Autodesk Inventor part; units mm, degrees
ref_plane "YZ Plane" through (0, 0, 0) normal (1, 0, 0) x (0, 1, 0)
ref_plane "XZ Plane" through (0, 0, 0) normal (0, 1, 0) x (-1, 0, 0)
ref_plane "XY Plane" through (0, 0, 0) normal (0, 0, 1) x (1, 0, 0)
sketch "스케치1" plane through (0, 0, 0) normal (0, 1, 0) x (-1, 0, 0)
  circle A0 centre (0, 0) radius 11
  circle A1 centre (0, -8) radius 1.1
  circle A2 centre (0, 0) radius 11
  circle A3 centre (8, 0) radius 1.1
  circle A4 centre (0, 0) radius 11
  circle A5 centre (0, 8) radius 1.1
  circle A6 centre (0, 0) radius 11
  circle A7 centre (-8, 0) radius 1.1
  line L0 (-11, 0) -> (-11, -150)
  line L1 (-11, -150) -> (11, -150)
  line L2 (11, -150) -> (11, 0)
  line L3 (16, -150) -> (-16, -150)
  line L4 (-16, -150) -> (-16, -50)
  line L5 (-16, -50) -> (16, -50)
  line L6 (16, -50) -> (16, -150)
  arc A8 (-11, 0) -> (11, 0) centre (0, 0) ccw
  circle A9 centre (0, 0) radius 4.5
  line L7 (25, -150) -> (-25, -150)
  line L8 (-25, -150) -> (-25, -60)
  line L9 (-25, -60) -> (25, -60)
  line L10 (25, -60) -> (25, -150)
  line L11 (16, -63.3333) -> (21, -63.3333)
  line L12 (21, -63.3333) -> (21, -103.3333)
  line L13 (21, -103.3333) -> (16, -103.3333)
  line L14 (16, -103.3333) -> (16, -63.3333)
  line L15 (16, -106.6667) -> (21, -106.6667)
  line L16 (21, -106.6667) -> (21, -146.6667)
  line L17 (21, -146.6667) -> (16, -146.6667)
  line L18 (16, -146.6667) -> (16, -106.6667)
  line L19 (-16, -63.3333) -> (-21, -63.3333)
  line L20 (-21, -63.3333) -> (-21, -103.3333)
  line L21 (-21, -103.3333) -> (-16, -103.3333)
  line L22 (-16, -103.3333) -> (-16, -63.3333)
  line L23 (-16, -106.6667) -> (-21, -106.6667)
  line L24 (-21, -106.6667) -> (-21, -146.6667)
  line L25 (-21, -146.6667) -> (-16, -146.6667)
  line L26 (-16, -146.6667) -> (-16, -106.6667)
  dimension "d1" = 2.2
  dimension "d5" = 360
  dimension "d7" = 150
  dimension "d8" = 32
  dimension "d9" = 100
  dimension "d24" = 9
  dimension "d26" = 50
  dimension "d27" = 90
  dimension "d28" = 9
  dimension "d29" = 5
  dimension "d30" = 40
  dimension "d31" = 5
  dimension "d32" = 40
  dimension "d33" = 3.3333
  dimension "d34" = 3.3333
  dimension "d35" = 5
  dimension "d36" = 40
  dimension "d37" = 5
  dimension "d38" = 40
  dimension "d39" = 3.3333
  dimension "d40" = 3.3333
extrude "돌출1" add sketch "스케치1" along normal blind 5 contours A0 | L2 L5 L0 A0 | L5 L6 L9 L2 | L2 L9 L0 L5 | L0 L9 L4 L5 | L9 L6 L3 L2 | L2 L1 L0 L9 | L0 L3 L4 L9 | L9 L10 L7 L6 L17 L16 L15 L13 L12 L11 | L4 L19 L20 L21 L23 L24 L25 L7 L8 L9
fillet "모깎기1" radius 2 18 edges at (16, 5, -83.3333) (16, 5, -126.6667) (16, 0, -126.6667) (16, 0, -83.3333) (-16, 5, -83.3333) (-16, 5, -126.6667) (16, 2.5, -50) (25, 2.5, -60) (16, 2.5, -60) (11, 2.5, -50) (-11, 2.5, -50) (-16, 2.5, -50) (-16, 2.5, -60) (-25, 2.5, -60) (-16, 0, -83.3333) (-16, 0, -126.6667) (25, 2.5, -150) (-25, 2.5, -150)
sketch "스케치2" plane through (0, 5, 0) normal (0, 1, 0) x (1, 0, 0)
  circle A0 centre (-8, 0) radius 1.1
  circle A1 centre (-8, 0) radius 2.1
  circle A2 centre (0, -8) radius 2.1
  circle A3 centre (8, 0) radius 2.1
  circle A4 centre (0, 8) radius 2.1
  point P0 (0, 0)
  dimension "d42" = 4.2
  dimension "d45" = 360
extrude "돌출2" cut sketch "스케치2" against normal blind 2
equation "\"d28\" = -0.5 * d8 + 0.5 * d26"
equation "\"d31\" = d29"
equation "\"d32\" = d30"
equation "\"d33\" = -0.333333 * d30 + 0.333333 * d27 - 0.333333 * d32"
equation "\"d34\" = -0.333333 * d30 + 0.333333 * d27 - 0.333333 * d32"
equation "\"d35\" = d29"
equation "\"d36\" = d30"
equation "\"d37\" = d29"
equation "\"d38\" = d30"
equation "\"d39\" = -0.333333 * d30 + 0.333333 * d27 - 0.333333 * d32"
equation "\"d40\" = -0.333333 * d30 + 0.333333 * d27 - 0.333333 * d32"
properties part number "arm2"
CAD build for the part. Positions are in the model's coordinates, mm. A direction names the side the tool comes from. Round coordinates to 2 decimals unless told otherwise and drop trailing zeros. Order: outer loops, then holes, each group sorted by start corner. A loop starts at its lowest first (then second) coordinate and runs counter-clockwise, first axis right, second up. Notation, with made-up numbers: (19.5, -9.75) -> (25.5, -9.75) arc R21 cw to (25.5, 16.25) -> close; hole circle Ø4 at (21, 64.25). An arc over 180 degrees is marked (long way). One line per question, with ' | ' between items.
Q1. Probe probe 1 along Z at (x, y) = (0, 4.05); probe 2 along Z at (x, y) = (0, 1.55); probe 3 along X at (y, z) = (2.85, -95). List the from-to ranges inside material, lowest first.
Completed:
probe 1: z = -150 to -10.1, -5.9 to -4.5, 4.5 to 5.9, 10.1 to 11 | probe 2: z = -150 to -9.1, -6.9 to -4.5, 4.5 to 6.9, 9.1 to 11 | probe 3: x = -25 to -21, -16 to 16, 21 to 25
Q2. Slice it at A-A (z = -42). Write the cut outline in (x, y), then the cut area to 3 significant figures.
Completed:
outline: (-11, 0) -> (11, 0) -> (11, 5) -> (-11, 5) -> close | area: 110 mm^2
Q3. Which spindle directions (+Z, -Z, +X, -X, +Y, -Y) get a long thin tool onto all of the face, cutting with end or side? Do faces 1 (the cylindrical face through (-0.273, 4.014, 5.918)), 2 (the cylindrical face through (0, 2, 11)), 3 (the flat face through (0, 0, -86)), 4 (the flat face through (-16, 2, -55)), 5 (the flat face through (21, 2, -60)). Say none if no direction does.
Completed:
face 1: +Y | face 2: +Z, +Y, -Y | face 3: +Z, -Z, +X, -X, -Y | face 4: +Z, -X, +Y, -Y | face 5: +Z, +X, +Y, -Y
Q4. Drop flat-ended pins along their axis: pin 1 (2.5 mm diameter, centred on x = -8, z = 0, fed in from +Y); pin 2 (0.5 mm diameter, centred on x = -13.5, y = 2, fed in from +Z); pin 3 (2.5 mm diameter, centred on x = -20, y = 3, fed in from +Z). Give the stop position or say it passes through.
Completed:
pin 1: stops at y = 3 | pin 2: stops at z = -50 | pin 3: stops at z = -60
Q5. Two-plate mould, pull along Z, no slides. Class faces 6 (the flat face through (16, 2, -55)), 7 (the flat face through (-20, 2, -60)), 8 (the cylindrical face through (-0.273, 4.014, -10.082)): released by +Z, released by -Z, zero draft, split by the parting line, or undercut.
Completed:
face 6: zero draft | face 7: released by +Z | face 8: undercut
